Print and shaded views of the part. All mm, measured from the part's lowest x, y and z. A direction names the side the tool comes from. Coordinates: 2 decimals unless noted, no trailing zeros. Loops run counter-clockwise (first coordinate to the right, second up) from the corner with the lowest first, then second, coordinate; pieces in that order, holes last. Notation, with made-up numbers: M 5,72 L 21,72 A21 cw 21,101 Z; hole C -6.75,10.5 d10. An arc over 180 degrees is marked long. One line per question, with ' | ' between items. Start each with the question number.
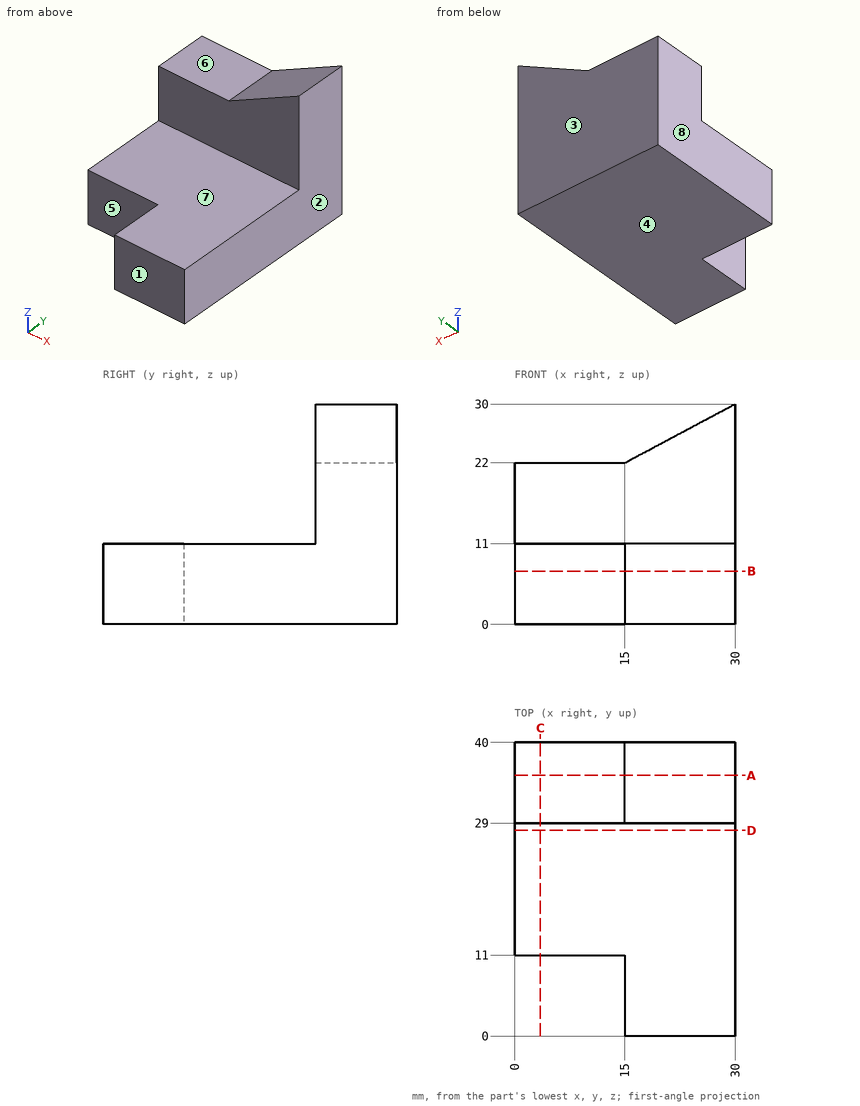
(1) Band-saw the part on C-C on x = 3.5. Write the cut outline in (y, z).
(2) Band-saw the part on D-D on y = 28. Write the cut outline in (x, z), then the cut area to 3 significant figures.
(3) Band-saw the part on B-B on z = 7.25. Write the cut outline in (x, y), then the cut area to 4 significant figures.
(4) Band-saw the part on A-A on y = 35.5. Write the cut outline in (x, z), then the cut area to 3 significant figures.
(5) Pin check, flat tips, straight feed: P1, Ø10, axis at x = 6.5, z = 10, coming from the -Y side; P2, Ø12, axis at x = 4.5, z = 26, coming from the -Y side; P3, Ø5.5, axis at x = 10, y = 36, coming from the +Z side; P4, Ø10, axis at y = 21.5, z = 25.5, coming from the +X side. Stop position of each tip, or through.
(6) Two-plate mould, pull along Y, no slides. Class the marked faces 1, 2 and 3: pulls with the +Y half, pulls with the -Y half, needs draft (parallel to the pull), parting line crosses it, or undercut.
(7) 3-axis set-ups, long thin cutter, end or side, ignore diameter. For the marked faces 4, 5, 6, 7 and 8: which of +Z, -Z, +X, -X, +Y, -Y reach the whole face in a straight line?
(8) Drill centre lines: line 1 (Z direction, x = 13.5, y = 27); line 2 (Y direction, x = 8.5, z = 4.75); line 3 (X direction, y = 10.5, z = 4.25). Where is each one in solid material? Low to high. Write a range as [from, to].
Computed values:
1) outline: M 11,0 L 40,0 L 40,22 L 29,22 L 29,11 L 11,11 Z
2) outline: M 0,0 L 30,0 L 30,11 L 0,11 Z | area: 330 mm^2
3) outline: M 0,11 L 15,11 L 15,0 L 30,0 L 30,40 L 0,40 Z | area: 1,035 mm^2
4) outline: M 0,0 L 30,0 L 30,30 L 15,22 L 0,22 Z | area: 720 mm^2
5) P1: y = 11 | P2: y = 29 | P3: z = 22 | P4: through
6) face 1: pulls with the -Y half | face 2: needs draft | face 3: pulls with the +Y half
7) face 4: -Z, +X, -X, +Y, -Y | face 5: +Z, -Z, -X, -Y | face 6: +Z, -X, +Y, -Y | face 7: +Z, +X, -X, -Y | face 8: +Z, -Z, -X, +Y, -Y
8) line 1: [0, 11] | line 2: [11, 40] | line 3: [15, 30]
